Read the model definition and answer for the solid it produces. Units are mm, in the model's axes. Coordinates: 2 decimals unless noted, no trailing zeros. Write each loop counter-clockwise with the first axis right and the second up, starting at its lowest first coordinate (ties: lowest second). Pieces come first, ordered by that corner, then holes. Notation, with made-up numbers: (41.25, -12.75) -> (94.25, -12.75) arc R26 cw to (94.25, 13.25) -> close; hole circle Ø11 at (7.5, -32). An arc over 180 degrees is marked (long way). Answer as a JSON object with one key per item and string values. Group by question number.
(1) Flat-ended cylindrical pins translate along their axes: P1, Ø6, axis at y = -6, z = 18.5, coming from the -X side; P2, Ø3, axis at x = -1, z = 18.5, coming from the +Y side; P3, Ø2, axis at y = 2.5, z = 27, coming from the -X side. Find the tip coordinate at first contact, or state that the pin passes through.
(2) Find section C-C (z = 18). Give the vertices of the cut face in (x, y), then the cut area to 3 significant figures.
(3) Find section A-A (y = 0). Give the vertices of the cut face in (x, z).
(4) Find section B-B (z = 3). Give the vertices of the cut face in (x, y).
(5) For a pull along Y with two mould halves and no side action, classify faces 1 (the face through (-1.08, -4.88, 29.63)), 2 (the face through (-4.4, -1.6, 0)), 3 (the face through (-0.59, -4.46, 9.86)) as +Y half, -Y half, draft (parallel to the pull), parting line (faces both ways), or undercut.
(6) Straight lines are drawn through the part: L1, parallel to X at y = 1.75, z = 10; L2, parallel to Y at x = 0.75, z = 10; L3, parallel to Y at x = 0.5, z = 4. For each, find the intervals that lie inside material, in ascending order.
(7) Find section D-D (z = 32). Give the vertices of the cut face in (x, y), then the cut area to 3 significant figures.
from build123d import *
from build123d import SkipClean  # not in build123d's __all__

# Parameters (mm, degrees)
F1_DEPTH = 20
F1_TAPER = 3
F3_DEPTH = 19
F3_TAPER = 3
F4_R     = 5
F5_DEPTH = 19
F6_R     = 4.5
F7_DEPTH = 20


with BuildPart() as f1:
    # F0 (on Top) → F1 (new body)
    with BuildSketch(Plane.XY):
        with BuildLine():
            ThreePointArc((-8.4714285714, -1.7482352618), (-7.3721516068, -2.5756206682), (-6.54, -3.6712940498))
            ThreePointArc((-6.54, -3.6712940498), (0, -7.5), (6.54, -3.6712940498))
            ThreePointArc((6.54, -3.6712940498), (7.3721516068, -2.5756206682), (8.4714285714, -1.7482352618))
            ThreePointArc((8.4714285714, -1.7482352618), (9.5, 0), (8.4714285714, 1.7482352618))
            ThreePointArc((8.4714285714, 1.7482352618), (7.3721516068, 2.5756206682), (6.54, 3.6712940498))
            ThreePointArc((6.54, 3.6712940498), (0, 7.5), (-6.54, 3.6712940498))
            ThreePointArc((-6.54, 3.6712940498), (-7.3721516068, 2.5756206682), (-8.4714285714, 1.7482352618))
            ThreePointArc((-8.4714285714, 1.7482352618), (-9.5, 0), (-8.4714285714, -1.7482352618))
        make_face()
    extrude(amount=F1_DEPTH, taper=F1_TAPER)

    # F2 (on face) → F3 (join)
    with BuildSketch(Plane.XY.offset(20)):
        with BuildLine():
            ThreePointArc((-5.6260083293, 3.1582157345), (-6.4518444143, 0), (-5.6260083293, -3.1582157345))
            ThreePointArc((-5.6260083293, -3.1582157345), (0, -6.4518444143), (5.6260083293, -3.1582157345))
            ThreePointArc((5.6260083293, -3.1582157345), (6.4518444143, 0), (5.6260083293, 3.1582157345))
            ThreePointArc((5.6260083293, 3.1582157345), (0, 6.4518444143), (-5.6260083293, 3.1582157345))
        make_face()
    with SkipClean():  # cleaning this boolean's faces spoils the solid; the shape is the same uncleaned
        extrude(amount=F3_DEPTH, taper=F3_TAPER)

    # F4 (on face) → F5 (cut)
    with BuildSketch(Plane.XY.offset(39)):
        Circle(F4_R)
    with SkipClean():  # cleaning this boolean's faces spoils the solid; the shape is the same uncleaned
        extrude(amount=-F5_DEPTH, mode=Mode.SUBTRACT)

    # F6 (on face) → F7 (cut, through all)
    with BuildSketch(Plane(origin=(0, 0, 0), x_dir=(1, 0, 0), z_dir=(0, 0, -1))):
        Circle(F6_R)
    with SkipClean():  # cleaning this boolean's faces spoils the solid; the shape is the same uncleaned
        extrude(amount=-F7_DEPTH, mode=Mode.SUBTRACT)


solid = f1.part
Results below:
{
 "1": {"P1": "stops at x = -5.82", "P2": "stops at y = 6.59", "P3": "stops at x = -5.9"},
 "2": {"outline": "(-8.01, -0.92) arc R5.94 cw to (-5.72, -3.21) arc R6.56 ccw to (5.72, -3.21) arc R5.94 cw to (8.01, -0.92) arc R1.06 ccw to (8.01, 0.92) arc R5.94 cw to (5.72, 3.21) arc R6.56 ccw to (-5.72, 3.21) arc R5.94 cw to (-8.01, 0.92) arc R1.06 ccw to start; hole circle Ø9 at (0, 0)", "area": "82.6 mm2"},
 "3": {"outline": "(-9.5, 0) -> (-4.5, 0) -> (-4.5, 20) -> (-5, 20) -> (-5, 39) -> (-5.46, 39) -> (-6.45, 20) -> (-8.45, 20) -> close; (4.5, 0) -> (9.5, 0) -> (8.45, 20) -> (6.45, 20) -> (5.46, 39) -> (5, 39) -> (5, 20) -> (4.5, 20) -> close"},
 "4": {"outline": "(-8.4, -1.61) arc R5.16 cw to (-6.4, -3.59) arc R7.34 ccw to (6.4, -3.59) arc R5.16 cw to (8.4, -1.61) arc R1.84 ccw to (8.4, 1.61) arc R5.16 cw to (6.4, 3.59) arc R7.34 ccw to (-6.4, 3.59) arc R5.16 cw to (-8.4, 1.61) arc R1.84 ccw to start; hole circle Ø9 at (0, 0)"},
 "5": {"face 1": "undercut", "face 2": "draft", "face 3": "undercut"},
 "6": {"L1": "x = -7.52 to -4.15, 4.15 to 7.52", "L2": "y = -6.94 to -4.44, 4.44 to 6.94", "L3": "y = -7.27 to -4.47, 4.47 to 7.27"},
 "7": {"outline": "circle Ø11.65 at (0, 0); hole circle Ø10 at (0, 0)", "area": "28.0 mm2"}
}
